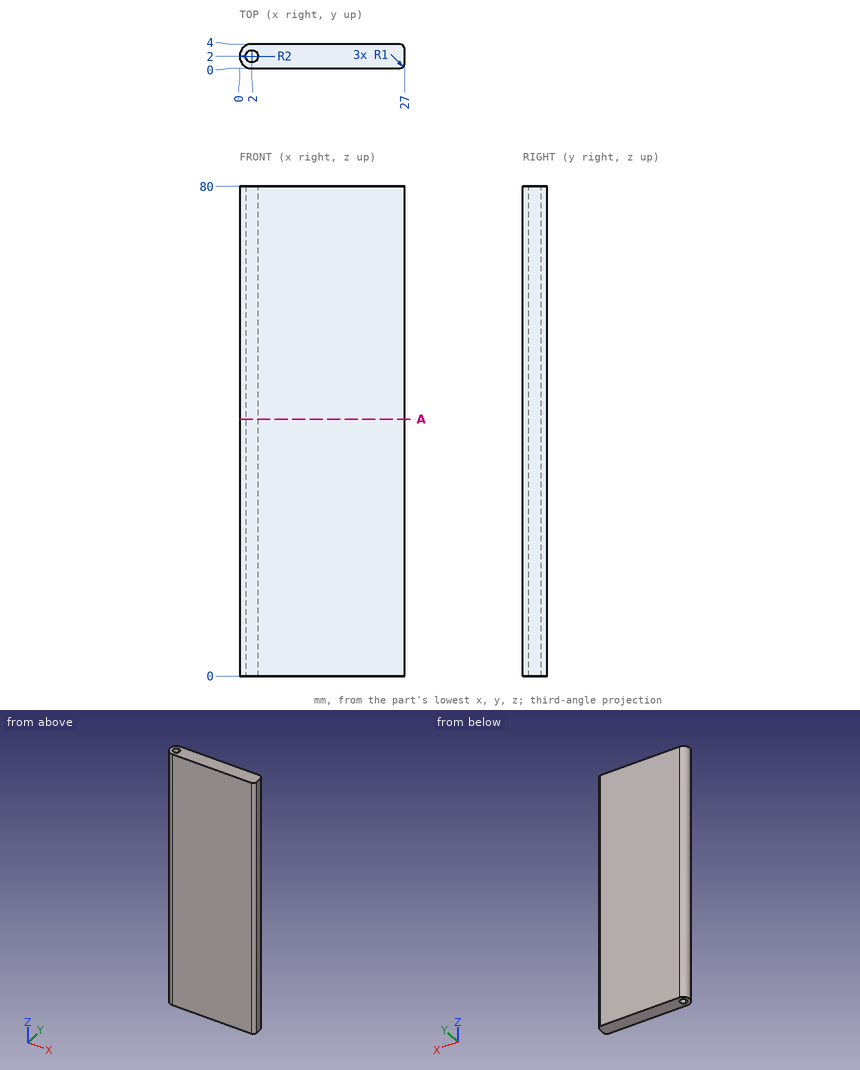
The figure shows three views and two pictorial views of one solid part (mm, origin at its lowest corner). Answer the questions. Coordinates: 2 decimals unless noted, no trailing zeros. Loops run counter-clockwise (first coordinate to the right, second up) from the corner with the lowest first, then second, coordinate; pieces in that order, holes last. Notation, with made-up numbers: (-19.75, -22.75) -> (26.25, -22.75) arc R11 cw to (26.25, -2.75) -> close; hole circle Ø7 at (-38.5, -37.5). An arc over 180 degrees is marked (long way). Return JSON: item names as keys, results as strings. Group by question number.
(1) Find the intervals of material crossed by probe 1 along X at (y, z) = (2.6, 38); probe 2 along X at (y, z) = (2.75, 37); probe 3 along X at (y, z) = (0.25, 27), in increasing order. Write a range as from..to.
(2) Given pin 1 Ø10 at (x, z) = (21.5, 24.5) entering from -Y, flat-ended and moving along its own axis, determine where the tip first touches the part or whether it passes through.
(3) A cutting plane is placed at A-A on z = 42. Write down the section's boundary in (x, y).
The answers:
{
 "1": {"probe 1": "x = 0.09..1.2, 2.8..27", "probe 2": "x = 0.15..1.34, 2.66..27", "probe 3": "x = 1.03..26.66"},
 "2": {"pin 1": "stops at y = 0"},
 "3": {"outline": "(2, 0) -> (26, 0) arc R1 ccw to (27, 1) -> (27, 3) arc R1 ccw to (26, 4) -> (2, 4) arc R2 ccw to start; hole circle Ø2 at (2, 2)"}
}
